The model under review builds one solid part; all positions refer to its coordinate system, in mm. A direction names the side the tool comes from. Round coordinates to 2 decimals unless told otherwise and drop trailing zeros. Order: outer loops, then holes, each group sorted by start corner. A loop starts at its lowest first (then second) coordinate and runs counter-clockwise, first axis right, second up. Notation, with made-up numbers: M -11.5,-10.75 L 0.5,-10.75 A5 ccw 0.5,-4.75 Z; hole C 58,-5.75 d1. An arc over 180 degrees is marked long. One line per item, written item: value. Start each with the question number.
from build123d import *

# Parameters (mm, degrees)
F0_W     = 550
F0_H     = 550
F1_DEPTH = 350
F2_W     = 530
F2_H     = 530
F3_DEPTH = 340


with BuildPart() as f1:
    # F0 (on Top) → F1 (new body)
    with BuildSketch(Plane.XY):
        with Locations((275, 275)):
            Rectangle(F0_W, F0_H)
    extrude(amount=-F1_DEPTH)

    # F2 (on Top) → F3 (cut)
    with BuildSketch(Plane.XY):
        with Locations((275, 275)):
            Rectangle(F2_W, F2_H)
    extrude(amount=-F3_DEPTH, mode=Mode.SUBTRACT)


solid = f1.part
Item 1: Consider section A-A, the plane z = -275. Give the boundary of the cut face in (x, y).
Item 2: Clearance check with a flat-ended pin moving along its axis: P1, Ø8, axis at x = 366, y = 150, coming from the +Z side. State where the tip first meets the part, or that it passes through.
Item 3: The part is to be moulded in two halves that separate along Y. For faces 1 (the flat face through (271, 0, -173)), 2 (the flat face through (271, 550, -173)), 3 (the flat face through (271, 10, -168)), say which applies: pulls with the +Y half, pulls with the -Y half, needs draft (parallel to the pull), parting line crosses it, or undercut.
Item 4: Wall thickness on L1, parallel to X at y = 214.5, z = -45; L2, parallel to Z at x = 219, y = 480.5: over which ranges is each line inside the solid? List them lowest first.
Item 5: Machinability: for faces 4 (the flat face through (271, 279, -350)), 5 (the flat face through (10, 271, -168)), which of the approach directions +Z, -Z, +X, -X, +Y, -Y give a long, thin tool a straight path to every point of the face, cutting with its end or side? Answer none if there is none.
Item 6: Consider section B-B, the plane x = 131. Give the boundary of the cut face in (y, z).
Computed:
1. outline: M 0,0 L 550,0 L 550,550 L 0,550 Z; hole M 10,10 L 540,10 L 540,540 L 10,540 Z
2. P1: stops at z = -340
3. face 1: pulls with the -Y half
3. face 2: pulls with the +Y half
3. face 3: undercut
4. L1: x = 0 to 10, 540 to 550
4. L2: z = -350 to -340
5. face 4: -Z, +X, -X, +Y, -Y
5. face 5: +Z
6. outline: M 0,-350 L 550,-350 L 550,0 L 540,0 L 540,-340 L 10,-340 L 10,0 L 0,0 Z
